```python
from build123d import *

# Parameters (mm, degrees)
SKETCH_3_R      = 1.8
SKETCH_3_W      = 0.8
SKETCH_3_H      = 1.5
SKETCH_3_W_2    = 1
EXTRUDE_2_DEPTH = 2


with BuildPart() as part:
    # 草图3 → 凸台-拉伸2 (new body)
    with BuildSketch(Plane(origin=(0, 0, 0), x_dir=(1, 0, 0), z_dir=(0, 1, 0))):
        with BuildLine():
            Line((8.65, -27), (8.65, -21.5))
            Line((8.65, -21.5), (8.65, -20))
            Line((8.65, -20), (1.9, -20))
            Line((1.9, -20), (-0.163508327, -20))
            ThreePointArc((-0.163508327, -20), (-2.1, -20.5), (-4.036491673, -20))
            Line((-4.036491673, -20), (-20, -20))
            Line((-20, -20), (-20, -5.443559577))
            ThreePointArc((-20, -5.443559577), (-20.4, -3.7), (-20, -1.956440423))
            Line((-20, -1.956440423), (-20, 6.361726266))
            ThreePointArc((-20, 6.361726266), (-23.3, 10.3), (-20, 14.238273734))
            Line((-20, 14.238273734), (-20, 20))
            Line((-20, 20), (-16.7, 20))
            Line((-16.7, 20), (-16.7, 27))
            Line((-16.7, 27), (-27, 27))
            Line((-27, 27), (-27, -27))
            Line((-27, -27), (8.65, -27))
        make_face()
        with Locations((-23.5, -23.5)):
            Circle(SKETCH_3_R, mode=Mode.SUBTRACT)
        with Locations((-23.5, 23.5)):
            Circle(SKETCH_3_R, mode=Mode.SUBTRACT)
        Polygon((20, -18), (20, -20), (20.65, -20), (20.65, -21.5), (20.65, -27), (27, -27), (27, 27), (-4.1, 27), (-4.1, 20), (20, 20), (20, -4), align=None)
        with Locations((23.5, -23.5)):
            Circle(SKETCH_3_R, mode=Mode.SUBTRACT)
        with Locations((23.5, 23.5)):
            Circle(SKETCH_3_R, mode=Mode.SUBTRACT)
        Polygon((12.4, -20), (12.4, -19.5), (12.4, -18), (10.4, -18), (1.9, -18), (1.9, -20), (8.65, -20), align=None)
        Polygon((20, -20), (16.9, -20), (16.9, -19.5), (16.1, -19.5), (13.4, -19.5), (12.4, -19.5), (12.4, -20), (8.65, -20), (8.65, -21.5), (20.65, -21.5), (20.65, -20), align=None)
        Polygon((16.9, -19.5), (16.9, -20), (20, -20), (20, -18), (16.9, -18), align=None)
        with Locations((16.5, -18.75)):
            Rectangle(SKETCH_3_W, SKETCH_3_H)
        with Locations((12.9, -18.75)):
            Rectangle(SKETCH_3_W_2, SKETCH_3_H)
        Polygon((16.1, -18), (16.9, -18), (16.9, -6), (12.4, -6), (12.4, -18), (13.4, -18), (13.4, -19.5), (16.1, -19.5), align=None)
        Polygon((16.9, -18), (20, -18), (20, -4), (10.4, -4), (10.4, -6), (10.4, -18), (12.4, -18), (12.4, -6), (16.9, -6), align=None)
    extrude(amount=EXTRUDE_2_DEPTH)


solid = part.part
```
Geometry: final body of the model. Coordinates: model frame, mm. A direction names the side the tool comes from. Coordinates: 2 decimals unless noted, no trailing zeros. Write each loop counter-clockwise with the first axis right and the second up, starting at its lowest first coordinate (ties: lowest second). Pieces come first, ordered by that corner, then holes. Notation, with made-up numbers: M 85,-30.75 L 115,-30.75 A26 ccw 115,-13.75 Z; hole C 78.5,-15 d8. An arc over 180 degrees is marked long. Answer as CSV lines item,"result". Start each with the question number.
Q1. Reachability of faces 4 (the flat face through (-16.7, 1, -23)), 5 (the flat face through (8.65, 1, 24)), 6 (the flat face through (1, 1, 20)) from +Z, -Z, +X, -X, +Y, -Y: full face, straight path, thin tool, end or side. Return the list, or none.
Q2. Pin query (flat end, axial travel): P1, Ø1, axis at x = 12.5, y = 1.5, coming from the +Z side. Return the tip coordinate at first contact, or that it passes through.
Q3. Mould query, pull axis X, two halves, no side actions, for faces 1 (the flat face through (27, 1, 0)), 2 (the flat face through (12, 1, -27)), 3 (the flat face through (10.4, 1, 11)). Classes: released by +X, released by -X, zero draft, split by the parting line, or undercut.
Q4. Cut plane C-C on y = 0.95. Count the separate pieces of the cut face and the enclosed holes in it, then the cut area to 3 significant figures.
Q5. Cut plane B-B on x = 13.5. Return the cut outline in (y, z).
Q6. Line query: line 1 (Z direction, x = -23.5, y = 1.15); line 2 (X direction, y = 1.4, z = 23.5); line 3 (Z direction, x = 15.5, y = 0.3). Output: solid intervals per line, ascending. Write a range as from..to.
Q7. Cut plane D-D on x = 23.5. Return the cut outline in (y, z), then the cut area to 3 significant figures.
Q8. Cut plane A-A on z = -3.5. Return the cut outline in (x, y), then the cut area to 3 significant figures.
Findings below:
1,face 4,"-Z, +Y, -Y"
1,face 5,"+Z, +Y, -Y"
1,face 6,"+Y, -Y"
2,P1,"stops at z = 21.5"
3,face 1,"released by +X"
3,face 2,"zero draft"
3,face 3,"undercut"
4,separate pieces,"1"
4,enclosed holes,"4"
4,area,"1,270 mm2"
5,outline,"M 0,-27 L 2,-27 L 2,-20 L 0,-20 Z; M 0,4 L 2,4 L 2,21.5 L 0,21.5 Z"
6,line 1,"z = -27..-25.3, -21.7..21.7, 25.3..27"
6,line 2,"x = -27..-25.3, -21.7..8.65, 20.65..21.7, 25.3..27"
6,line 3,"z = -27..-20, 4..21.5"
7,outline,"M 0,-27 L 2,-27 L 2,-25.3 L 0,-25.3 Z; M 0,-21.7 L 2,-21.7 L 2,21.7 L 0,21.7 Z; M 0,25.3 L 2,25.3 L 2,27 L 0,27 Z"
7,area,"93.6 mm2"
8,outline,"M -27,0 L -20,0 L -20,2 L -27,2 Z; M 20,0 L 27,0 L 27,2 L 20,2 Z"
8,area,"28.0 mm2"
